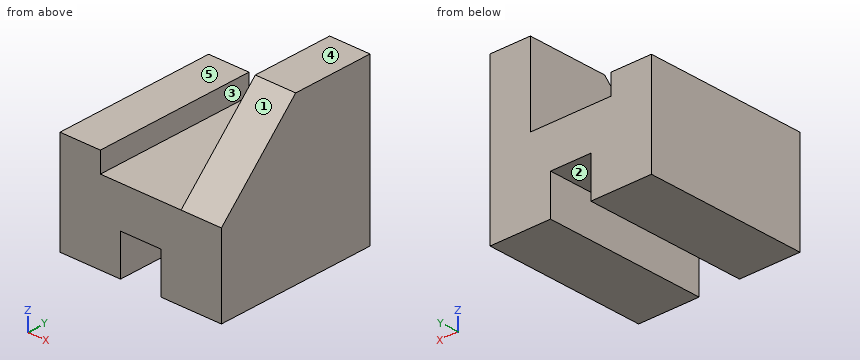
```python
from build123d import *

# Parameters (mm, degrees)
F1_DEPTH = 101.6
F3_DEPTH = 25.4


with BuildPart() as f1:
    # F0 (on Front) → F1 (new body)
    with BuildSketch(Plane.XZ):
        Polygon((-38.1, 0), (0, 0), (0, 101.6), (-25.4, 101.6), (-25.4, 50.8), (-76.2, 50.8), (-76.2, 63.5), (-101.6, 63.5), (-101.6, 0), (-63.5, 0), (-63.5, 25.4), (-38.1, 25.4), align=None)
    extrude(amount=F1_DEPTH)

    # F2 (on face) → F3 (cut)
    with BuildSketch(Plane.YZ):
        Polygon((-101.6, 101.6), (-101.6, 50.8), (-50.8, 101.6), align=None)
    extrude(amount=-F3_DEPTH, mode=Mode.SUBTRACT)


solid = f1.part
```
Source: CAD feature listing. Evaluate the final solid. Frame: model axes, mm. Face numbers are marked on the shaded views. A direction names the side the tool comes from. Coordinates: 2 decimals unless noted, no trailing zeros. Loops run counter-clockwise (first coordinate to the right, second up) from the corner with the lowest first, then second, coordinate; pieces in that order, holes last. Notation, with made-up numbers: M 2.5,58.5 L 45.5,58.5 A13 cw 45.5,79.5 Z; hole C 78,48.25 d6. An arc over 180 degrees is marked long. Put each result on its own line as item: value. Start each with the question number.
1) Ray query, L1, parallel to X at y = -17, z = 56.5; L2, parallel to Z at x = -41, y = -33; L3, parallel to X at y = -93, z = 18. Return the intervals inside material, ascending. Write a range as from..to.
2) Cut plane D-D on x = -8.5. Return the cut outline in (y, z).
3) Contact query for flat-ended pins moving along their axis: pin 1 Ø3 at (x, z) = (-81, 26.5) entering from +Y; pin 2 Ø20.5 at (x, y) = (-95, -44) entering from +Z; pin 3 Ø1 at (x, y) = (-63.5, -23.5) entering from +Z; pin 4 Ø8 at (x, z) = (-53, 58.5) entering from +Y. Output: stop coordinate, or through.
4) Cut plane C-C on z = 21. Return the cut outline in (x, y), then the cut area to 3 significant figures.
5) Reachability of the marked faces 1, 2, 3, 4 and 5 from +Z, -Z, +X, -X, +Y, -Y: full face, straight path, thin tool, end or side. Return the list, or none.
6) Cut plane A-A on z = 61. Return the cut outline in (x, y).
7) Cut plane B-B on y = -93.5. Return the cut outline in (x, z), then the cut area to 3 significant figures.
The answers:
1. L1: x = -101.6..-76.2, -25.4..0
1. L2: z = 25.4..50.8
1. L3: x = -101.6..-63.5, -38.1..0
2. outline: M -101.6,0 L 0,0 L 0,101.6 L -50.8,101.6 L -101.6,50.8 Z
3. pin 1: stops at y = 0
3. pin 2: stops at z = 63.5
3. pin 3: stops at z = 50.8
3. pin 4: passes through
4. outline: M -101.6,-101.6 L -63.5,-101.6 L -63.5,0 L -101.6,0 Z; M -38.1,-101.6 L 0,-101.6 L 0,0 L -38.1,0 Z
4. area: 7,740 mm²
5. face 1: +Z, +X, -Y
5. face 2: -Z, +Y, -Y
5. face 3: +Z, +Y, -Y
5. face 4: +Z, +X, -X, +Y, -Y
5. face 5: +Z, -X, +Y, -Y
6. outline: M -101.6,-101.6 L -76.2,-101.6 L -76.2,0 L -101.6,0 Z; M -25.4,-91.4 L 0,-91.4 L 0,0 L -25.4,0 Z
7. outline: M -101.6,0 L -63.5,0 L -63.5,25.4 L -38.1,25.4 L -38.1,0 L 0,0 L 0,58.9 L -25.4,58.9 L -25.4,50.8 L -76.2,50.8 L -76.2,63.5 L -101.6,63.5 Z
7. area: 5,040 mm²
